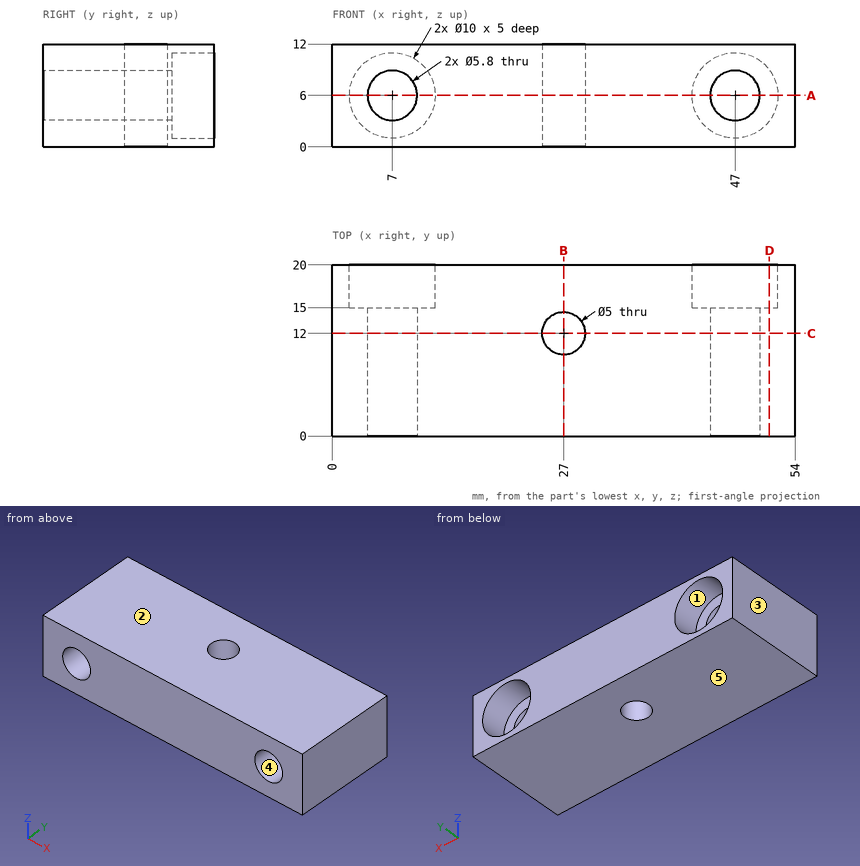
Here's the drawing with two shaded views (mm, measured from the low corner). I have some questions. A direction names the side the tool comes from. Round coordinates to 2 decimals unless told otherwise and drop trailing zeros. Loops run counter-clockwise (first coordinate to the right, second up) from the corner with the lowest first, then second, coordinate; pieces in that order, holes last. Notation, with made-up numbers: M 69,-22 L 94,-22 A25 cw 94,14 Z; hole C 54.5,56 d3. An arc over 180 degrees is marked long. Put each result on its own line as item: value.
Q1. Thinking about a two-plate mould opening in X: for the marked faces 3, 4 and 5, which applies, released by +X, released by -X, zero draft, split by the parting line, or undercut?
Check result:
face 3: released by -X
face 4: undercut
face 5: zero draft
Q2. Imagine slicing it at A-A (z = 6). Write out the boundary of the cut face in (x, y), then the cut area to 3 significant figures.
Check result:
outline: M 0,0 L 4.1,0 L 4.1,15 L 2,15 L 2,20 L 0,20 Z; M 9.9,0 L 44.1,0 L 44.1,15 L 42,15 L 42,20 L 12,20 L 12,15 L 9.9,15 Z; M 49.9,0 L 54,0 L 54,20 L 52,20 L 52,15 L 49.9,15 Z; hole C 27,12 d5
area: 786 mm2
Q3. Imagine slicing it at C-C (y = 12). Write out the boundary of the cut face in (x, z), then the cut area to 3 significant figures.
Check result:
outline: M 0,0 L 24.5,0 L 24.5,12 L 0,12 Z; M 29.5,0 L 54,0 L 54,12 L 29.5,12 Z; hole C 7,6 d5.8; hole C 47,6 d5.8
area: 535 mm2
Q4. On a 3-axis mill with a long thin cutter (end or side, diameter ignored), from which of +Z, -Z, +X, -X, +Y, -Y can I reach the whole of each face in a straight line? I mean the marked faces 1 and 2. Say none if no direction works.
Check result:
face 1: +Y
face 2: +Z, +X, -X, +Y, -Y
Q5. For pin 1 (3 mm diameter, centred on x = 7.5, z = 4.5, fed in from +Y); pin 2 (4.5 mm diameter, centred on x = 27, y = 12, fed in from +Z), each with a flat end and sliding along its axis, tell me the tip position at first contact or that it passes through.
Check result:
pin 1: y = 15
pin 2: through
Q6. Imagine slicing it at B-B (x = 27). Write out the boundary of the cut face in (y, z), then the cut area to 3 significant figures.
Check result:
outline: M 0,0 L 9.5,0 L 9.5,12 L 0,12 Z; M 14.5,0 L 20,0 L 20,12 L 14.5,12 Z
area: 180 mm2
Q7. I need wall thicknesses on probe 1 along Z at (x, y) = (7, 4.5); probe 2 along Y at (x, z) = (27, 5.25); probe 3 along X at (y, z) = (18.75, 7.5). Which ranges of each line are inside material? Lowest first, please.
Check result:
probe 1: 0 to 3.1, 8.9 to 12
probe 2: 0 to 9.5, 14.5 to 20
probe 3: 0 to 2.23, 11.77 to 42.23, 51.77 to 54
Q8. Imagine slicing it at D-D (x = 51). Write out the boundary of the cut face in (y, z).
Check result:
outline: M 0,0 L 20,0 L 20,3 L 15,3 L 15,9 L 20,9 L 20,12 L 0,12 Z
